Verification items for this drawing (mm, ordinates from the low corner). Coordinates: 2 decimals unless noted, no trailing zeros. Loops run counter-clockwise (first coordinate to the right, second up) from the corner with the lowest first, then second, coordinate; pieces in that order, holes last. Notation, with made-up numbers: M 5.25,-11.5 L 17.25,-11.5 A31 ccw 17.25,27.5 Z; hole C 22.25,-39.5 d3. An arc over 180 degrees is marked long. Return JSON: item names as keys, results as strings.
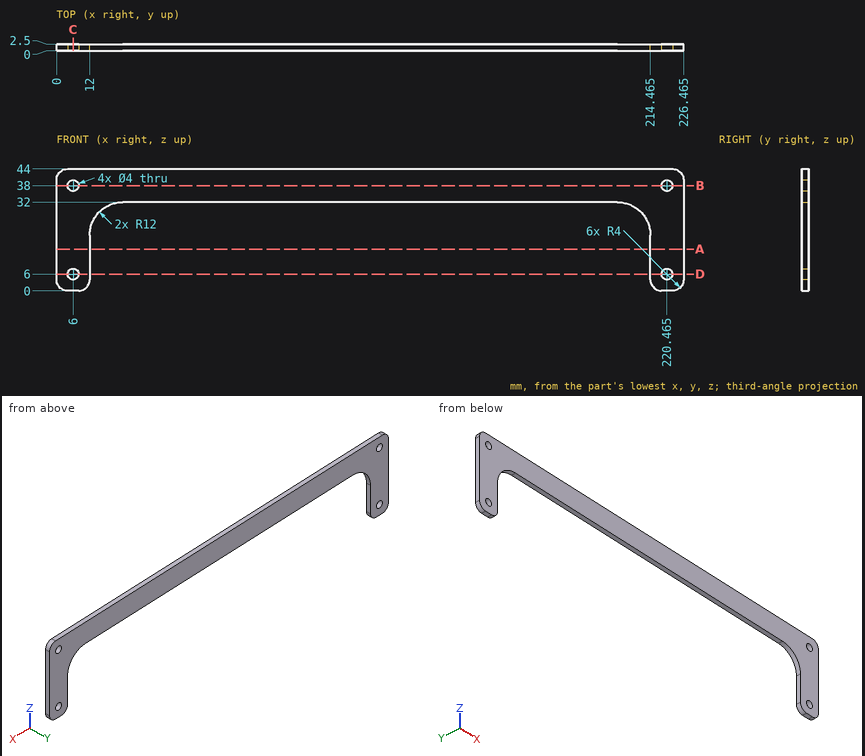
1) Section check A-A on z = 15. Record the cut outline in (x, y) (1 decimal).
Answers:
{"outline": "M 0,0 L 12,0 L 12,2.5 L 0,2.5 Z; M 214.5,0 L 226.5,0 L 226.5,2.5 L 214.5,2.5 Z"}
2) Section check B-B on z = 38. Record the cut outline in (x, y) (1 decimal).
Answers:
{"outline": "M 0,0 L 4,0 L 4,2.5 L 0,2.5 Z; M 8,0 L 218.5,0 L 218.5,2.5 L 8,2.5 Z; M 222.5,0 L 226.5,0 L 226.5,2.5 L 222.5,2.5 Z"}
3) Section check D-D on z = 6. Record the cut outline in (x, y) (1 decimal), then the cut area to 3 significant figures.
Answers:
{"outline": "M 0,0 L 4,0 L 4,2.5 L 0,2.5 Z; M 8,0 L 12,0 L 12,2.5 L 8,2.5 Z; M 214.5,0 L 218.5,0 L 218.5,2.5 L 214.5,2.5 Z; M 222.5,0 L 226.5,0 L 226.5,2.5 L 222.5,2.5 Z", "area": "40.0 mm²"}
4) Section check C-C on x = 6. Record the cut outline in (y, z).
Answers:
{"outline": "M 0,0 L 2.5,0 L 2.5,4 L 0,4 Z; M 0,8 L 2.5,8 L 2.5,36 L 0,36 Z; M 0,40 L 2.5,40 L 2.5,44 L 0,44 Z"}
5) Go/stop test with flat-tipped pins: pin 1 Ø12 at (x, z) = (31.5, 25) entering from +Y; pin 2 Ø0.8 at (x, y) = (99.5, 1) entering from -Z. Record where each tip stops, or that it passes through.
Answers:
{"pin 1": "through", "pin 2": "z = 32"}
6) Scan lines: line 1 along X through (y, z) = (0.5, 6) (1 decimal); line 2 along X through (y, z) = (1.7, 38) (1 decimal); line 3 along X through (y, z) = (1, 14) (1 decimal). Record each from-to range of solid material in increasing order. Write a range as [from, to].
Answers:
{"line 1": "[0, 4], [8, 12], [214.5, 218.5], [222.5, 226.5]", "line 2": "[0, 4], [8, 218.5], [222.5, 226.5]", "line 3": "[0, 12], [214.5, 226.5]"}
